Autodesk Inventor part; units mm, degrees
ref_plane "YZ Plane" through (0, 0, 0) normal (1, 0, 0) x (0, 1, 0)
ref_plane "XZ Plane" through (0, 0, 0) normal (0, 1, 0) x (-1, 0, 0)
ref_plane "XY Plane" through (0, 0, 0) normal (0, 0, 1) x (1, 0, 0)
sketch "Sketch1" plane through (0, 0, 0) normal (0, 1, 0) x (-1, 0, 0)
  line L0 (-17.6, 0) -> (-17.6, -17.6)
  line L1 (-17.6, -17.6) -> (0, -17.6)
  line L2 (17.6, 0) -> (17.6, -17.6)
  line L3 (17.6, -17.6) -> (0, -17.6)
  line L4 (-17.6, 0) -> (-17.6, 17.6)
  line L5 (-17.6, 17.6) -> (0, 17.6)
  line L6 (17.6, 17.6) -> (0, 17.6)
  line L7 (17.6, 0) -> (17.6, 17.6)
  point P0 (0, 0)
  dimension "d0" = 17.6
  dimension "d1" = 17.6
extrude "Extrusion1" add sketch "Sketch1" along normal blind 28.2
sketch "Sketch2" plane through (0, 28.2, 0) normal (0, 1, 0) x (1, 0, 0)
  circle A0 centre (13, 13) radius 1.5
  circle A1 centre (-13, 13) radius 1.5
  circle A2 centre (13, -13) radius 1.5
  circle A3 centre (-13, -13) radius 1.5
  point P0 (0, 0)
  dimension "d4" = 3
  dimension "d5" = 3
  dimension "d6" = 3
  dimension "d7" = 3
extrude "Extrusion2" cut sketch "Sketch2" against normal blind 4.5
chamfer "Chamfer1" distance 3 angle 45 4 edges at (17.6, 14.1, 17.6) (17.6, 14.1, -17.6) (-17.6, 14.1, 17.6) (-17.6, 14.1, -17.6)
sketch "Sketch3" plane through (0, 28.2, 0) normal (0, 1, 0) x (1, 0, 0)
  circle A0 centre (0, 0) radius 11
  dimension "d13" = 22
extrude "Extrusion3" add sketch "Sketch3" along normal blind 2
sketch "Sketch4" plane through (0, 30.2, 0) normal (0, 1, 0) x (1, 0, 0)
  circle A0 centre (0, 0) radius 2.5
  dimension "d16" = 5
extrude "Extrusion4" add sketch "Sketch4" along normal blind 22
chamfer "Chamfer2" distance 0.5 angle 45 1 edges at (-2.5, 52.2, 0)
properties part number "14HM11"
Verification items for the finished model (mm, model axes). A direction names the side the tool comes from. Give positions to 0.01 mm unless a question says otherwise; leave off trailing zeros. Loops run counter-clockwise (first coordinate to the right, second up) from the corner with the lowest first, then second, coordinate; pieces in that order, holes last. Notation, with made-up numbers: (52.25, 51.5) - (76.25, 51.5) arc R19 ccw to (76.25, 86.5) - close; hole circle Ø1 at (-15, 69.5). An arc over 180 degrees is marked (long way). Write each question's results on one line, items separated by ' | '.
1) Sectioned sample at D-D on x = -13. Record the boundary of the cut face in (y, z), plus the area to 3 significant figures.
Solution:
outline: (0, -17.6) - (28.2, -17.6) - (28.2, -14.5) - (23.7, -14.5) - (23.7, -11.5) - (28.2, -11.5) - (28.2, 11.5) - (23.7, 11.5) - (23.7, 14.5) - (28.2, 14.5) - (28.2, 17.6) - (0, 17.6) - close | area: 966 mm2
2) Tool access check on faces 5 (the flat face through (13, 23.7, -13)), 6 (the flat face through (-16.1, 14.3, -16.1)). Record the directions out of +Z, -Z, +X, -X, +Y, -Y that give a thin tool (end or side, any length) a straight path to the whole face; none if there is none.
Solution:
face 5: +Y | face 6: -Z, -X, +Y, -Y
3) Sectioned sample at B-B on x = 0. Record the boundary of the cut face in (y, z), plus the area to 3 significant figures.
Solution:
outline: (0, -17.6) - (28.2, -17.6) - (28.2, -11) - (30.2, -11) - (30.2, -2.5) - (51.7, -2.5) - (52.2, -2) - (52.2, 2) - (51.7, 2.5) - (30.2, 2.5) - (30.2, 11) - (28.2, 11) - (28.2, 17.6) - (0, 17.6) - close | area: 1,150 mm2
4) Sectioned sample at C-C on y = 36. Record the boundary of the cut face in (x, z), plus the area to 3 significant figures.
Solution:
outline: circle Ø5 at (0, 0) | area: 19.6 mm2
5) Mould release check, pull along X, two halves, no side actions. Record for faces 1 (the cylindrical face through (11.5, 25.98, 12.93)), 2 (the flat face through (8, 28.2, -8)), 3 (the cylindrical face through (-0.54, 40.8, -2.44)), 4 (the flat face through (-13, 23.7, -13)): pulls with the +X half, pulls with the -X half, needs draft (parallel to the pull), parting line crosses it, or undercut.
Solution:
face 1: undercut | face 2: needs draft | face 3: parting line crosses it | face 4: undercut
6) Sectioned sample at A-A on z = 13. Record the boundary of the cut face in (x, y), plus the area to 3 significant figures.
Solution:
outline: (-17.6, 0) - (17.6, 0) - (17.6, 28.2) - (14.5, 28.2) - (14.5, 23.7) - (11.5, 23.7) - (11.5, 28.2) - (-11.5, 28.2) - (-11.5, 23.7) - (-14.5, 23.7) - (-14.5, 28.2) - (-17.6, 28.2) - close | area: 966 mm2
7) Depth check by flat-ended pin: P1, Ø3.5, axis at x = -13, z = -12.5, coming from the +Y side; P2, Ø0.9, axis at x = 12.5, z = -13.5, coming from the +Y side; P3, Ø4, axis at x = 7, y = 32, coming from the -Z side. Enter the tip coordinate at first touch or a pass-through.
Solution:
P1: y = 28.2 | P2: y = 23.7 | P3: z = -9.13
8) Material ranges on L1, parallel to Z at x = 13, y = 26.3; L2, parallel to Y at x = -12.5, z = 3, recorded low to high. Write a range as from..to.
Solution:
L1: -17.6..-14.5, -11.5..11.5, 14.5..17.6 | L2: 0..28.2
